CAD build for the part. Positions are in the model's coordinates, mm. A direction names the side the tool comes from. Coordinates: 2 decimals unless noted, no trailing zeros. Loops run counter-clockwise (first coordinate to the right, second up) from the corner with the lowest first, then second, coordinate; pieces in that order, holes last. Notation, with made-up numbers: (15.25, 63) -> (54.25, 63) arc R9 cw to (54.25, 72) -> close; hole circle Ø8 at (78, -13.75). An arc over 180 degrees is marked (long way). Write each question's results on one line, items separated by ' | '.
```python
from build123d import *

# Parameters (mm, degrees)
BOSS_EXTRUDE1_DEPTH = 5
SKETCH3_R           = 4
CUT_EXTRUDE1_DEPTH  = 5


with BuildPart() as part:
    # Sketch1 → Boss-Extrude1 (new body)
    with BuildSketch(Plane.XY):
        with BuildLine():
            Line((-38.916331436, -113.987341772), (0, -95))
            Line((0, -95), (38.916331436, -113.987341772))
            ThreePointArc((38.916331436, -113.987341772), (51.961524227, -110), (48.8920671, -96.708860759))
            Line((48.8920671, -96.708860759), (12.990381057, -72.5))
            Line((12.990381057, -72.5), (9.991552325, 0.410952718))
            Line((9.991552325, 0.410952718), (10, 30))
            ThreePointArc((10, 30), (0, 40), (-10, 30))
            Line((-10, 30), (-9.991552325, 0.410952718))
            Line((-9.991552325, 0.410952718), (-12.990381057, -72.5))
            Line((-12.990381057, -72.5), (-48.8920671, -96.708860759))
            ThreePointArc((-48.8920671, -96.708860759), (-51.961524227, -110), (-38.916331436, -113.987341772))
        make_face()
    extrude(amount=BOSS_EXTRUDE1_DEPTH)

    # Sketch3 → Cut-Extrude1 (cut)
    with BuildSketch(Plane(origin=(0, 0, 0), x_dir=(-1, 0, 0), z_dir=(0, 0, -1))):
        with Locations((0, 30)):
            Circle(SKETCH3_R)
        Circle(SKETCH3_R)
    extrude(amount=-CUT_EXTRUDE1_DEPTH, mode=Mode.SUBTRACT)


solid = part.part
```
Q1. Cut at D-D on y = -67. Write the cut outline in (x, z).
Results are:
outline: (-12.76, 0) -> (12.76, 0) -> (12.76, 5) -> (-12.76, 5) -> close
Q2. Pull direction Y, two halves, no side cores. Call faces 3 (the cylindrical face through (0.867, -3.905, 2.465)), 4 (the cylindrical face through (0, 40, 2)), 5 (the cylindrical face through (-52.065, -109.817, 2.465)): +Y half, -Y half, draft (parallel to the pull), parting line (faces both ways), or undercut.
Results are:
face 3: undercut | face 4: +Y half | face 5: parting line
Q3. Drop flat-ended pins along their axis: pin 1 (3 mm diameter, centred on y = 1.5, z = 2, fed in from -X); pin 2 (1 mm diameter, centred on x = -41, y = -89.5, fed in from -Z); pin 3 (1 mm diameter, centred on x = 21, z = 3, fed in from -Y); pin 4 (2.5 mm diameter, centred on y = 13.5, z = 2.5, fed in from +X). Give the stop position or say it passes through.
Results are:
pin 1: x = -10.01 | pin 2: through | pin 3: y = -105.49 | pin 4: x = 10
Q4. Cut at B-B on y = -105. Write the cut outline in (x, z), and give its area (3 significant figures).
Results are:
outline: (-53.3, 0) -> (-20.5, 0) -> (-20.5, 5) -> (-53.3, 5) -> close; (20.5, 0) -> (53.3, 0) -> (53.3, 5) -> (20.5, 5) -> close | area: 328 mm^2
Q5. Wall check: L1, parallel to Y at x = 0, z = 2.2; L2, parallel to Y at x = 2.5, z = 2.8; L3, parallel to X at y = 12, z = 4.35. Give the ranges that are in metal, low to high. Write a range as from..to.
Results are:
L1: -95..-4, 4..26, 34..40 | L2: -96.22..-3.12, 3.12..26.88, 33.12..39.68 | L3: -9.99..9.99
Q6. Cut at A-A on z = 3.9. Write the cut outline in (x, y), and give its area (3 significant figures).
Results are:
outline: (-48.89, -96.71) arc R10 ccw to (-38.92, -113.99) -> (0, -95) -> (38.92, -113.99) arc R10 ccw to (48.89, -96.71) -> (12.99, -72.5) -> (9.99, 0.41) -> (10, 30) arc R10 ccw to (-10, 30) -> (-9.99, 0.41) -> (-12.99, -72.5) -> close; hole circle Ø8 at (0, 0); hole circle Ø8 at (0, 30) | area: 4,890 mm^2
Q7. Cut at C-C on x = 27.5. Write the cut outline in (y, z).
Results are:
outline: (-108.42, 0) -> (-82.28, 0) -> (-82.28, 5) -> (-108.42, 5) -> close
Q8. Which spindle directions (+Z, -Z, +X, -X, +Y, -Y) get a long thin tool onto all of the face, cutting with end or side? Do faces 1 (the flat face through (31.19, -84.77, 2.46)), 2 (the flat face through (-19.731, -104.627, 2.465)). Say none if no direction does.
Results are:
face 1: +Z, -Z, +X, +Y | face 2: +Z, -Z, -Y
